Autodesk Inventor part; units mm, degrees
ref_plane "YZ Plane" through (0, 0, 0) normal (1, 0, 0) x (0, 1, 0)
ref_plane "XZ Plane" through (0, 0, 0) normal (0, 1, 0) x (-1, 0, 0)
ref_plane "XY Plane" through (0, 0, 0) normal (0, 0, 1) x (1, 0, 0)
sketch "Sketch1" plane through (0, 0, 0) normal (0, 0, 1) x (1, 0, 0)
  line L0 (0, 0) -> (20, 0)
  line L1 (20, 0) -> (20, 22.2)
  line L2 (20, 22.2) -> (0, 22.2)
  line L3 (0, 22.2) -> (0, 0)
  dimension "d0" = 20
  dimension "d1" = 22.2
extrude "Extrusion1" add sketch "Sketch1" along normal mid plane 11.8
sketch "Sketch2" plane through (0, 0, 5.9) normal (-1, 0, 0) x (0, 0, 1)
  circle A0 centre (-5.9, 5.9) radius 5.9
  line L0 (0, 0) -> (-11.8, 0)
  line L1 (0, 22.2) -> (0, 0)
  point P0 (-5.9, 0)
  dimension "d4" = 5.9
  dimension "d5" = 5.9
  dimension "d6" = 11.8
extrude "Extrusion2" add sketch "Sketch2" along normal blind 3 contours A0
sketch "Sketch3" plane through (0, 22.2, 5.9) normal (0, 1, 0) x (1, 0, 0)
  line L0 (0, 0) -> (20, 0)
  line L1 (3, 11.6) -> (4.3, 11.6)
  line L2 (4.3, 11.6) -> (4.3, 0)
  line L3 (4.3, 0) -> (3, 0)
  line L4 (3, 0) -> (3, 11.6)
  line L5 (0, 11.8) -> (0, 0)
  point P0 (0, 5.9)
  dimension "d9" = 3
  dimension "d10" = 1.3
  dimension "d11" = 11.6
extrude "Extrusion3" add sketch "Sketch3" along normal blind 5 and the other way blind 27.2
properties part number "Servo"
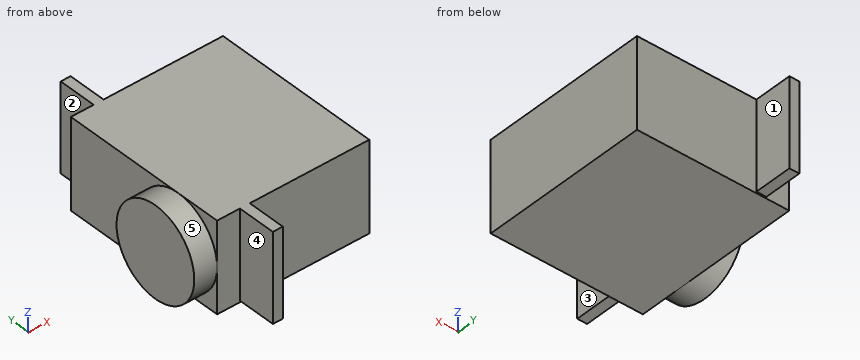
The listing builds one solid part. Answer for the finished solid, in the listing's coordinates (mm). Face numbers are marked on the shaded views. A direction names the side the tool comes from. Give positions to 0.01 mm unless a question says otherwise; leave off trailing zeros. Write each loop counter-clockwise with the first axis right and the second up, starting at its lowest first coordinate (ties: lowest second). Pieces come first, ordered by that corner, then holes. Notation, with made-up numbers: (-33.75, 15) - (-18.75, 15) arc R17 ccw to (-18.75, 23) - close; hole circle Ø11 at (73.25, -30.75). An arc over 180 degrees is marked (long way). Use a Markdown table: item, result.
1. Section A-A on y = -1.5 is taken. Write down the section's boundary in (x, z).
Values follow:
| item | result |
|---|---|
| outline | (3, -5.7) - (4.3, -5.7) - (4.3, 5.9) - (3, 5.9) - close |
2. A tool of negligible diameter and unlimited length cuts with its end or side. For the marked faces 1, 2, 3, 4 and 5, from which of +Z, -Z, +X, -X, +Y, -Y can it reach the whole face along a straight path? Write none if from no direction.
Values follow:
| item | result |
|---|---|
| face 1 | +Z, -Z, +X, +Y |
| face 2 | +Z, -Z, -X, +Y |
| face 3 | +Z, -Z, +X, -Y |
| face 4 | +Z, -Z, -X, -Y |
| face 5 | -X |
3. Section C-C on z = -5 is taken. Write down the section's boundary in (x, y), plus the area to 3 significant figures.
Values follow:
| item | result |
|---|---|
| outline | (-3, 2.77) - (0, 2.77) - (0, 0) - (3, 0) - (3, -5) - (4.3, -5) - (4.3, 0) - (20, 0) - (20, 22.2) - (4.3, 22.2) - (4.3, 27.2) - (3, 27.2) - (3, 22.2) - (0, 22.2) - (0, 9.03) - (-3, 9.03) - close |
| area | 476 mm² |
4. Section B-B on x = 8.75 is taken. Write down the section's boundary in (y, z), plus the area to 3 significant figures.
Values follow:
| item | result |
|---|---|
| outline | (0, -5.9) - (22.2, -5.9) - (22.2, 5.9) - (0, 5.9) - close |
| area | 262 mm² |
5. Each of these flat-tipped pins is pushed along its axis until it touches: P1, Ø1, axis at x = 3.5, y = -2, coming from the -Z side; P2, Ø3, axis at x = 11, z = -2.5, coming from the +Y side; P3, Ø3.5, axis at x = 8.5, z = 1, coming from the -Y side. Where does it stop, or does it pass through?
Values follow:
| item | result |
|---|---|
| P1 | stops at z = -5.7 |
| P2 | stops at y = 22.2 |
| P3 | stops at y = 0 |
6. Find the intervals of material crossed by probe 1 along X at (y, z) = (-4, -3.25); probe 2 along Y at (x, z) = (15.25, 4.25); probe 3 along X at (y, z) = (17, 5.75), in increasing order. Write a range as from..to.
Values follow:
| item | result |
|---|---|
| probe 1 | x = 3..4.3 |
| probe 2 | y = 0..22.2 |
| probe 3 | x = 0..20 |
